Here's how the part is built. I have some questions about the finished solid (model axes, mm). Face numbers are marked on the shaded views. A direction names the side the tool comes from. Give positions to 0.01 mm unless a question says otherwise; leave off trailing zeros. Order: outer loops, then holes, each group sorted by start corner. A loop starts at its lowest first (then second) coordinate and runs counter-clockwise, first axis right, second up. Notation, with made-up numbers: M 77,83.5 L 91,83.5 A10 ccw 91,87.5 Z; hole C 18,0.5 d6. An arc over 180 degrees is marked long. One line per item, written item: value. Start each with the question number.
Autodesk Inventor part; units mm, degrees
ref_plane "YZ Plane" through (0, 0, 0) normal (1, 0, 0) x (0, 1, 0)
ref_plane "XZ Plane" through (0, 0, 0) normal (0, 1, 0) x (-1, 0, 0)
ref_plane "XY Plane" through (0, 0, 0) normal (0, 0, 1) x (1, 0, 0)
sketch "Sketch1" plane through (0, 0, 0) normal (0, 1, 0) x (-1, 0, 0)
  line L0 (0, 0) -> (19.05, 0)
  line L1 (19.05, 0) -> (19.05, -25.4)
  line L2 (19.05, -25.4) -> (0, -25.4)
  line L3 (0, -25.4) -> (0, 0)
  dimension "d0" = 25.4
  dimension "d1" = 19.05
extrude "Plate1" add sketch "Sketch1" along normal blind 3.048
sketch "Sketch2" plane through (-19.05, 3.048, -3.048) normal (0, 0, 1) x (1, 0, 0)
  line L0 (19.05, 0) -> (0, 0)
  line L1 (0, 0) -> (0, -31.75)
  line L2 (0, -31.75) -> (19.05, -31.75)
  line L3 (19.05, -31.75) -> (19.05, 0)
edge flange "Flange1" height 31.75 angle 90 thickness 3.048 bend radius 3.048 thickness toward (0, 0, 1) relief tear relief width 3.048 relief depth 1.524 edges at (-9.525, 0, 0) wall of the first edge with corners at (0, 3.048, -3.048) (-19.05, 3.048, -3.048) (-19.05, -28.702, -3.048) (0, -28.702, -3.048)
bend "Bend1"
corner "Corner1"
sketch "Sketch3" plane through (0, 3.048, 0) normal (0, 1, 0) x (1, 0, 0)
  line L0 (-19.05, 6.096) -> (-19.05, 25.4)
  line L1 (-19.05, 25.4) -> (0, 25.4)
  circle A0 centre (-9.525, 15.748) radius 5.5563
  point P0 (0, 0)
  dimension "d13" = 11.1125
extrude "Cut1" cut sketch "Sketch3" against normal blind 3.048
fillet "Corner Round1" radius 9.525 2 edges at (0, 1.524, -25.4) (-19.05, 1.524, -25.4)
sketch "Sketch5" plane through (-19.05, -28.702, 0) normal (0, 0, 1) x (1, 0, 0)
  line L0 (0, 0) -> (0, 25.654)
  line L1 (19.05, 0) -> (0, 0)
  line L2 (19.05, 25.654) -> (19.05, 0)
  line L3 (19.05, 25.654) -> (0, 25.654)
  line L4 (0, 25.654) -> (19.05, 25.654)
  line L5 (9.525, 25.654) -> (9.525, 17.1027)
  line L6 (9.525, 17.1027) -> (9.525, 8.5429)
  circle A0 centre (9.525, 17.1027) radius 3.175
  circle A1 centre (9.525, 8.5429) radius 3.175
  point P0 (19.05, 28.702)
  dimension "d17" = 8.5513
  dimension "d18" = 8.5598
  dimension "d19" = 6.35
  dimension "d20" = 6.35
extrude "Cut2" cut sketch "Sketch5" against normal blind 3.048 contours A0 L6 L5 | L5 L6 A0 | A1
equation "\"d14\" = Thickness"
equation "\"d21\" = Thickness"
equation "\"d3\" = BendReliefWidth"
equation "\"d4\" = BendReliefDepth"
equation "\"d5\" = MinimumRemnant"
equation "\"d6\" = BendRadius"
equation "\"d9\" = BendRadius"
equation "\"d10\" = CornerReliefSize"
equation "\"d11\" = GapSize"
equation "\"d12\" = JacobiRadiusSize"
equation "\"BendRadius\" = Thickness"
equation "\"BendReliefWidth\" = Thickness"
equation "\"BendReliefDepth\" = 0.5 * Thickness"
equation "\"CornerReliefSize\" = 4 * Thickness"
equation "\"MinimumRemnant\" = 2 * Thickness"
equation "\"TransitionRadius\" = BendRadius"
equation "\"JacobiRadiusSize\" = BendRadius"
equation "\"GapSize\" = Thickness"
equation "\"d2\" = BendRadius"
properties part number "RSL plate"
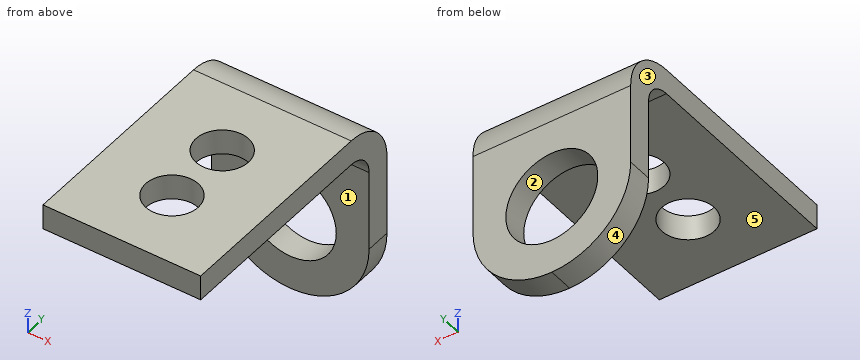
Item 1: I want a section at C-C on z = -20. Write out the boundary of the cut face in (x, y).
Item 2: I want a section at A-A on x = -12.25. Write out the boundary of the cut face in (y, z).
Item 3: Please list where these lines run through material, in increasing order: probe 1 along Y at (x, z) = (-17.25, -11.5); probe 2 along Z at (x, y) = (-5.25, -15.5); probe 3 along X at (y, z) = (2, -14). Write a range as [from, to].
Item 4: We'd pull the mould along X, two halves only. Please class the marked faces 1, 2 and 3: +X half, -X half, draft (parallel to the pull), parting line (faces both ways), or undercut.
Item 5: For the marked faces 4 and 5, which set-ups out of +Z, -Z, +X, -X, +Y, -Y let a thin tool reach every point of the face, with its end or its side?
Item 6: I want a section at B-B on y = -21. Write out the boundary of the cut face in (x, z).
Item 7: Will these pins go through, and if not, where does the flat tip stop? P1, Ø8, axis at x = -11.5, z = -8.5, coming from the -Y side; P2, Ø1.5, axis at x = -4, z = -9, coming from the -Y side; P3, Ø5, axis at x = -6.5, y = -11, coming from the -Z side; P4, Ø5, axis at x = -9.52, y = -11.6, coming from the -Z side.
Answer below:
1. outline: M -18.11,0 L -13.1,0 L -13.1,3.05 L -18.11,3.05 Z; M -5.95,0 L -0.94,0 L -0.94,3.05 L -5.95,3.05 Z
2. outline: M -28.7,-3.05 L -21.79,-3.05 L -21.79,0 L -28.7,0 Z; M -18.53,-3.05 L -13.23,-3.05 L -13.23,0 L -18.53,0 Z; M -9.97,-3.05 L -3.05,-3.05 A3.05 cw 0,-6.1 L 0,-10.91 L 3.05,-10.91 L 3.05,-6.1 A6.1 ccw -3.05,0 L -9.97,0 Z; M 0,-25 L 3.05,-25 L 3.05,-20.59 L 0,-20.59 Z
3. probe 1: y = [0, 3.05]
3. probe 2: z = [-3.05, 0]
3. probe 3: x = [-19.05, -14.8], [-4.25, 0]
4. face 1: draft
4. face 2: undercut
4. face 3: -X half
5. face 4: -Z, -X, +Y, -Y
5. face 5: -Z, +X, -X, -Y
6. outline: M -19.05,-3.05 L -12.59,-3.05 L -12.59,0 L -19.05,0 Z; M -6.46,-3.05 L 0,-3.05 L 0,0 L -6.46,0 Z
7. P1: stops at y = -0.45
7. P2: stops at y = 0
7. P3: stops at z = -3.05
7. P4: passes through
